For this review, take the finished solid that the model builds, in its own axes (mm). A direction names the side the tool comes from. Coordinates: 2 decimals unless noted, no trailing zeros. Loops run counter-clockwise (first coordinate to the right, second up) from the corner with the lowest first, then second, coordinate; pieces in that order, holes last. Notation, with made-up numbers: M -24,64.25 L -6,64.25 A19 ccw -6,76.25 Z; hole C 74,34.25 d2. An arc over 180 degrees is marked long. Write item = value, one per line.
from build123d import *

# Parameters (mm, degrees)
SKETCH1_W           = 55.88
SKETCH1_H           = 63.5
BOSS_EXTRUDE1_DEPTH = 25.4
FILLET1_R           = 2
BOSS_EXTRUDE2_DEPTH = 25.4


with BuildPart() as part:
    # Sketch1 → Boss-Extrude1 (new body)
    with BuildSketch(Plane.XY):
        with Locations((27.94, 31.75)):
            Rectangle(SKETCH1_W, SKETCH1_H)
    extrude(amount=BOSS_EXTRUDE1_DEPTH)

    # Fillet1
    fillet1_edges = [part.edges().sort_by_distance(p)[0] for p in [
        (55.88, 31.75, 25.4),
        (27.94, 63.5, 25.4),
        (0, 31.75, 25.4),
        (27.94, 63.5, 0),
        (55.88, 31.75, 0),
        (27.94, 0, 0),
        (0, 31.75, 0),
        (27.94, 0, 25.4),
        (0, 63.5, 12.7),
        (55.88, 63.5, 12.7),
        (55.88, 0, 12.7),
        (0, 0, 12.7),
    ]]
    fillet(fillet1_edges, radius=FILLET1_R)

    # Sketch3 → Boss-Extrude2 (add)
    with BuildSketch(Plane.ZY.offset(-15)):
        with BuildLine():
            Line((25.4, 61.5), (25.4, 59.5))
            ThreePointArc((25.4, 59.5), (29.4, 55.5), (25.4, 51.5))
            Line((25.4, 51.5), (25.4, 49.5))
            ThreePointArc((25.4, 49.5), (28.228427125, 48.328427125), (29.4, 45.5))
            Line((29.4, 45.5), (29.4, 1.05))
            ThreePointArc((29.4, 1.05), (28.2, -0.15), (27, 1.05))
            ThreePointArc((27, 1.05), (26.25, 1.8), (25.5, 1.05))
            ThreePointArc((25.5, 1.05), (28.2, -1.65), (30.9, 1.05))
            Line((30.9, 1.05), (30.9, 55.5))
            ThreePointArc((30.9, 55.5), (29.316951072, 59.569705149), (25.4, 61.5))
        make_face()
    extrude(amount=-BOSS_EXTRUDE2_DEPTH)


solid = part.part
Q1. For pin 1 Ø6 at (x, z) = (33, 4.5) entering from -Y; pin 2 Ø1.5 at (y, z) = (27, 24.5) entering from +X; pin 3 Ø3 at (y, z) = (34, 28) entering from -X, all flat-tipped, find the tip position at first contact; note any pin that passes through.
Solved:
pin_1 = 0
pin_2 = 55.85
pin_3 = 15
Q2. Draft analysis for pull direction Y (two halves, no side actions). For faces 4 (the face through (28, 32, 0)), 5 (the face through (55.28, 0.57, 12.85)), 6 (the face through (28, 24, 29.4)), state which applies: +Y half, -Y half, draft (parallel to the pull), parting line (faces both ways), or undercut.
Solved:
face_4 = draft
face_5 = -Y half
face_6 = undercut
Q3. Add section B-B (z = 5). Write out the cut boundary in (x, y), and give its area (3 significant figures).
Solved:
outline = M 0,2 A2 ccw 2,0 L 53.88,0 A2 ccw 55.88,2 L 55.88,61.5 A2 ccw 53.88,63.5 L 2,63.5 A2 ccw 0,61.5 Z
area = 3,540 mm²
Q4. Add section C-C (x = 5). Write out the cut boundary in (y, z), and give its area (3 significant figures).
Solved:
outline = M 0,2 A2 ccw 2,0 L 61.5,0 A2 ccw 63.5,2 L 63.5,23.4 A2 ccw 61.5,25.4 L 2,25.4 A2 ccw 0,23.4 Z
area = 1,610 mm²
Q5. For line 1 along Z through (x, y) = (20.5, 31); line 2 along Y through (x, z) = (43, 22.5); line 3 along Z through (x, y) = (10.5, 13), list the stretches that pass through material, from the lowest coordinate up.
Solved:
line_1 = 0 to 25.4, 29.4 to 30.9
line_2 = 0 to 63.5
line_3 = 0 to 25.4
Q6. Add section A-A (y = 32.5). Write out the cut boundary in (x, z), and give its area (3 significant figures).
Solved:
outline = M 0,2 A2 ccw 2,0 L 53.88,0 A2 ccw 55.88,2 L 55.88,23.4 A2 ccw 53.88,25.4 L 2,25.4 A2 ccw 0,23.4 Z; M 15,29.4 L 40.4,29.4 L 40.4,30.9 L 15,30.9 Z
area = 1,450 mm²
Q7. Add section D-D (z = 28.2). Write out the cut boundary in (x, y).
Solved:
outline = M 15,-1.65 L 40.4,-1.65 L 40.4,-0.15 L 15,-0.15 Z; M 15,48.36 L 40.4,48.36 L 40.4,52.64 L 15,52.64 Z; M 15,58.36 L 40.4,58.36 L 40.4,60.52 L 15,60.52 Z
Q8. Machinability: for faces 1 (the face through (15, 32, 30)), 2 (the face through (27.5, 1.8, 26.3)), 3 (the face through (40.4, 32, 30)), which of the approach directions +Z, -Z, +X, -X, +Y, -Y give a long, thin tool a straight path to every point of the face, cutting with its end or side? Answer none if there is none.
Solved:
face_1 = +Z, -X, +Y, -Y
face_2 = +X, -X
face_3 = +Z, +X, +Y, -Y
